Autodesk Inventor part; units mm, degrees
ref_plane "YZ Plane" through (0, 0, 0) normal (1, 0, 0) x (0, 1, 0)
ref_plane "XZ Plane" through (0, 0, 0) normal (0, 1, 0) x (-1, 0, 0)
ref_plane "XY Plane" through (0, 0, 0) normal (0, 0, 1) x (1, 0, 0)
sketch "Sketch1" plane through (0, 0, 0) normal (1, 0, 0) x (0, 1, 0)
  line L0 (0, 0) -> (16, 0)
  line L1 (16, 0) -> (16, -100)
  line L2 (16, -100) -> (0, -100)
  line L3 (0, -10) -> (0, -10)
  line L4 (0, -10) -> (0, -25)
  line L5 (0, -25) -> (0, -25)
  line L6 (0, -90) -> (0, -90)
  line L7 (0, -90) -> (0, -75)
  line L8 (0, -75) -> (0, -75)
  line L9 (0, -10) -> (0, 0)
  line L10 (0, -100) -> (0, -90)
  line L11 (0, -75) -> (0, -25)
  dimension "d0" = 16
  dimension "d1" = 100
  dimension "d2" = 0
  dimension "d3" = 15
  dimension "d4" = 10
  dimension "d5" = 15
  dimension "d6" = 10
  dimension "d10" = 0
  dimension "d11" = 0
  dimension "d12" = 0
extrude "Extrusion1" add sketch "Sketch1" along normal blind 2
sketch "Sketch3" plane through (2, 0, 0) normal (1, 0, 0) x (0, 0, -1)
  circle A0 centre (10, 8) radius 2.5
  circle A1 centre (32, 8) radius 2.5
  circle A2 centre (44, 8) radius 2.5
  line L0 (0, 16) -> (0, 0)
  line L1 (100, 16) -> (0, 16)
  circle A3 centre (56, 8) radius 2.5
  dimension "d18" = 5
  dimension "d19" = 5
  dimension "d20" = 5
  dimension "d21" = 10
  dimension "d22" = 8
  dimension "d23" = 8
  dimension "d24" = 22
  dimension "d25" = 8
  dimension "d26" = 12
  dimension "d29" = 5
  dimension "d31" = 8
  dimension "d32" = 12
extrude "Extrusion3" cut sketch "Sketch3" against normal blind 10 contours A0 | A1 | A2
extrude "Extrusion4" cut sketch "Sketch3" against normal blind 10 contours A3
sketch "Sketch5" plane through (2, 0, 0) normal (1, 0, 0) x (0, 0, -1)
  line L0 (0, 0) -> (100, 0)
  circle A0 centre (63.5, -19) radius 2.5
  line L1 (56.5, 0) -> (72.5, 0)
  line L2 (72.5, 0) -> (72.5, -25)
  line L3 (72.5, -25) -> (56.5, -25)
  line L4 (56.5, -25) -> (56.5, 0)
  circle A1 centre (66.2831, 1.8148) radius 2.5
  circle A2 centre (56, 8) radius 6 construction
  circle A3 centre (63.5, -19) radius 15 construction
  circle A4 centre (66.2831, 1.8148) radius 6 construction
  dimension "d44" = 16
  dimension "d45" = 25
  dimension "d46" = 9
  dimension "d52" = 5
  dimension "d56" = 12
  dimension "d57" = 30
  dimension "d58" = 12
extrude "Extrusion6" add sketch "Sketch5" against normal blind 2 contours L0 A1 L2 L3 L4 | L0 A1 picked at (65.8534, -0.1091)
sketch "Sketch6" plane through (2, 0, 0) normal (1, 0, 0) x (0, 0, -1)
  circle A0 centre (66.2831, 1.8148) radius 2.5
  circle A1 centre (66.2831, 1.8148) radius 2.5
  point P0 (0, 0)
  dimension "d53" = 5
extrude "Extrusion7" cut sketch "Sketch6" against normal blind 3
properties part number "Mounting_wall_2"
For this review, take the finished solid that the model builds, in its own axes (mm). A direction names the side the tool comes from. Give positions to 0.01 mm unless a question says otherwise; leave off trailing zeros. Write each loop counter-clockwise with the first axis right and the second up, starting at its lowest first coordinate (ties: lowest second). Pieces come first, ordered by that corner, then holes. Notation, with made-up numbers: M 54.25,47.25 L 95.25,47.25 A25 ccw 95.25,81.25 Z; hole C 44.25,21.5 d10. An arc over 180 degrees is marked long. Answer as a JSON object with one key per item and string values. Group by question number.
Item 1: Consider section B-B on z = -10. Write out the cut boundary in (x, y), plus the area to 3 significant figures.
Item 2: Tool access review of faces 1 (the cylindrical face through (1.014, -18.249, -65.885)), 2 (the flat face through (1, -12, -72.5)), 3 (the flat face through (1, 0, -29)): name each direction out of +Z, -Z, +X, -X, +Y, -Y from which nothing blocks a thin tool from reaching the whole face with its end or side.
Item 3: Draft analysis for pull direction Z (two halves, no side actions). For faces 4 (the cylindrical face through (1.01, 7.04, -46.31)), 5 (the flat face through (1, -13, -56.5)), 6 (the flat face through (1, 16, -49)), state which applies: +Z half, -Z half, draft (parallel to the pull), parting line (faces both ways), or undercut.
Item 4: Consider section A-A on y = 8. Write out the cut boundary in (x, z).
Item 5: Consider section C-C on y = -19. Write out the cut boundary in (x, z).
Item 6: For pin 1 Ø6.5 at (y, z) = (-19, -63.5) entering from -X; pin 2 Ø0.6 at (x, y) = (0.5, -7.5) entering from +Z; pin 3 Ø0.6 at (x, y) = (0.5, -13) entering from -Z; pin 4 Ø10 at (y, z) = (-5.5, -30) entering from +X, all flat-tipped, find the tip position at first contact; note any pin that passes through.
Item 7: Consider section D-D on x = 0.9. Write out the cut boundary in (y, z).
Item 8: For probe 1 along Z at (x, y) = (1.7, 2); probe 2 along Y at (x, z) = (0.9, -10); probe 3 along Z at (x, y) = (0.7, -20), list the stretches that pass through material, from the lowest coordinate up. Write a range as [from, to].
Check result:
{
 "1": {"outline": "M 0,0 L 2,0 L 2,5.5 L 0,5.5 Z; M 0,10.5 L 2,10.5 L 2,16 L 0,16 Z", "area": "22.0 mm^2"},
 "2": {"face 1": "+X, -X", "face 2": "-Z, +X, -X, -Y", "face 3": "+Z, +X, -X, -Y"},
 "3": {"face 4": "undercut", "face 5": "+Z half", "face 6": "draft"},
 "4": {"outline": "M 0,-100 L 2,-100 L 2,-58.5 L 0,-58.5 Z; M 0,-53.5 L 2,-53.5 L 2,-46.5 L 0,-46.5 Z; M 0,-41.5 L 2,-41.5 L 2,-34.5 L 0,-34.5 Z; M 0,-29.5 L 2,-29.5 L 2,-12.5 L 0,-12.5 Z; M 0,-7.5 L 2,-7.5 L 2,0 L 0,0 Z"},
 "5": {"outline": "M 0,-72.5 L 2,-72.5 L 2,-66 L 0,-66 Z; M 0,-61 L 2,-61 L 2,-56.5 L 0,-56.5 Z"},
 "6": {"pin 1": "stops at x = 0", "pin 2": "stops at z = -56.5", "pin 3": "stops at z = -72.5", "pin 4": "passes through"},
 "7": {"outline": "M -25,-72.5 L 0,-72.5 L 0,-100 L 16,-100 L 16,0 L 0,0 L 0,-56.5 L -25,-56.5 Z; hole C -19,-63.5 d5; hole C 1.81,-66.28 d5; hole C 8,-56 d5; hole C 8,-44 d5; hole C 8,-32 d5; hole C 8,-10 d5"},
 "8": {"probe 1": "z = [-100, -68.78], [-63.79, 0]", "probe 2": "y = [0, 5.5], [10.5, 16]", "probe 3": "z = [-72.5, -65.79], [-61.21, -56.5]"}
}
